```python
from build123d import *

# Parameters (mm, degrees)
BOSS_EXTRUDE1_DEPTH  = 50
M4_CLEARANCE_HOLE1_D = 4.8


with BuildPart() as part:
    # Sketch1 → Boss-Extrude1 (new body)
    with BuildSketch(Plane(origin=(0, 0, 0), x_dir=(1, 0, 0), z_dir=(0, 1, 0))):
        with BuildLine():
            Line((-1.5875, -2.749630657), (-1.5875, -22.749630657))
            Line((-1.5875, -22.749630657), (-5.5875, -22.749630657))
            Line((-5.5875, -22.749630657), (-5.5875, -4.501163044))
            ThreePointArc((-5.5875, -4.501163044), (0, 7.175), (5.5875, -4.501163044))
            Line((5.5875, -4.501163044), (5.5875, -22.749630657))
            Line((5.5875, -22.749630657), (1.5875, -22.749630657))
            Line((1.5875, -22.749630657), (1.5875, -2.749630657))
            ThreePointArc((1.5875, -2.749630657), (3.175, 0), (1.5875, 2.749630657))
            Line((1.5875, 2.749630657), (-1.5875, 2.749630657))
            ThreePointArc((-1.5875, 2.749630657), (-3.175, 0), (-1.5875, -2.749630657))
        make_face()
    extrude(amount=BOSS_EXTRUDE1_DEPTH)

    # M4 Clearance Hole1 (through all)
    with Locations(Plane(origin=(5.5875, 0, 0), x_dir=(0, 0, -1), z_dir=(1, 0, 0))):
        with Locations((-15.249630657, 40), (-15.249630657, 10)):
            Hole(M4_CLEARANCE_HOLE1_D / 2)


solid = part.part
```
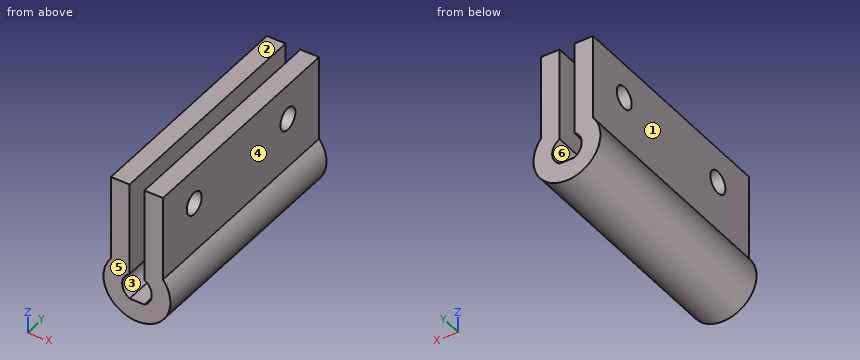
Geometry: final body of the model. Coordinates: model frame, mm. Face numbers are marked on the shaded views. A direction names the side the tool comes from. Coordinates: 2 decimals unless noted, no trailing zeros. Order: outer loops, then holes, each group sorted by start corner. A loop starts at its lowest first (then second) coordinate and runs counter-clockwise, first axis right, second up. Notation, with made-up numbers: M 89,8.25 L 116,8.25 A20 ccw 116,21.25 Z; hole C 52.25,17.25 d11. An arc over 180 degrees is marked long. Answer in a Markdown table with one row per item. Add a question column.
Q1. Mould query, pull axis X, two halves, no side actions, for the marked faces 1, 2 and 3. Classes: released by +X, released by -X, zero draft, split by the parting line, or undercut.
Q2. Section query C-C on z = 14. Return the cut outline in (x, y), and give its area (3 significant figures).
Q3. Line query: L1, parallel to X at y = 42.5, z = 15.25; L2, parallel to Y at x = 5.25, z = 15.5; L3, parallel to Z at x = -4.5, y = 6. Output: solid intervals per line, ascending.
Q4. Reachability of the marked faces 4, 5 and 6 from +Z, -Z, +X, -X, +Y, -Y: full face, straight path, thin tool, end or side. Return the list, or none.
Q5. Section query D-D on x = 4.5. Return the cut outline in (y, z).
Q6. Contact query for flat-ended pins moving along their axis: P1, Ø5, axis at x = 5, y = 42.5, coming from the -Z side; P2, Ø7.5, axis at y = 10, z = 15.25, coming from the -X side; P3, Ø3, axis at y = 28.5, z = 11.5, coming from the +X side; P4, Ø6, axis at x = 1, y = 32.5, coming from the +Z side. Output: stop coordinate, or through.
Q7. Section query A-A on y = 10. Count the separate pieces of the cut face and the enclosed holes in it, and give its area (3 significant figures).
Q8. Section query B-B on z = 0. Return the cut outline in (x, y) (3 decimals).
Completed:
| question | item | result |
|---|---|---|
| 1 | face 1 | released by -X |
| 1 | face 2 | zero draft |
| 1 | face 3 | undercut |
| 2 | outline | M -5.59,0 L -1.59,0 L -1.59,7.95 L -5.59,7.95 Z; M -5.59,12.05 L -1.59,12.05 L -1.59,37.95 L -5.59,37.95 Z; M -5.59,42.05 L -1.59,42.05 L -1.59,50 L -5.59,50 Z; M 1.59,0 L 5.59,0 L 5.59,7.95 L 1.59,7.95 Z; M 1.59,12.05 L 5.59,12.05 L 5.59,37.95 L 1.59,37.95 Z; M 1.59,42.05 L 5.59,42.05 L 5.59,50 L 1.59,50 Z |
| 2 | area | 334 mm2 |
| 3 | L1 | x = -5.59 to -1.59, 1.59 to 5.59 |
| 3 | L2 | y = 0 to 7.61, 12.39 to 37.61, 42.39 to 50 |
| 3 | L3 | z = -5.59 to 22.75 |
| 4 | face 4 | +Z, +X, +Y, -Y |
| 4 | face 5 | +Z, -Z, +X, -X, -Y |
| 4 | face 6 | +Y, -Y |
| 5 | outline | M 0,-5.59 L 50,-5.59 L 50,22.75 L 0,22.75 Z; hole C 10,15.25 d4.8; hole C 40,15.25 d4.8 |
| 6 | P1 | stops at z = -6.73 |
| 6 | P2 | stops at x = -5.59 |
| 6 | P3 | stops at x = 5.59 |
| 6 | P4 | stops at z = 22.75 |
| 7 | separate pieces | 3 |
| 7 | enclosed holes | 0 |
| 7 | area | 213 mm2 |
| 8 | outline | M -7.175,0 L -3.175,0 L -3.175,50 L -7.175,50 Z; M 3.175,0 L 7.175,0 L 7.175,50 L 3.175,50 Z |
